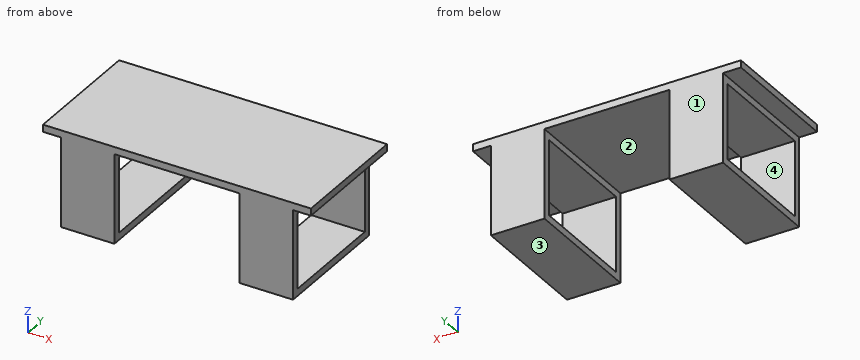
from build123d import *

# Parameters (mm, degrees)
F0_W     = 1500
F0_H     = 700
F1_DEPTH = 40
F2_W     = 300
F2_H     = 700
F3_DEPTH = 500
F4_W     = 620
F4_H     = 420
F5_DEPTH = 1328


with BuildPart() as f1:
    # F0 (on Top) → F1 (new body)
    with BuildSketch(Plane.XY):
        with Locations((750, -350)):
            Rectangle(F0_W, F0_H)
    extrude(amount=-F1_DEPTH)

    # F2 (on face) → F3 (join)
    with BuildSketch(Plane(origin=(0, 0, -40), x_dir=(1, 0, 0), z_dir=(0, 0, -1))):
        with Locations((250, 350)):
            Rectangle(F2_W, F2_H)
        with Locations((1250, 350)):
            Rectangle(F2_W, F2_H)
    extrude(amount=F3_DEPTH)

    # F4 (on face) → F5 (cut)
    with BuildSketch(Plane(origin=(100, 0, 0), x_dir=(0, -1, 0), z_dir=(-1, 0, 0))):
        with Locations((350, -290)):
            Rectangle(F4_W, F4_H)
    extrude(amount=-F5_DEPTH, mode=Mode.SUBTRACT)


solid = f1.part
Read the model definition and answer for the solid it produces. Units are mm, in the model's axes. Face numbers are marked on the shaded views. A direction names the side the tool comes from. Round coordinates to 2 decimals unless told otherwise and drop trailing zeros. Write each loop counter-clockwise with the first axis right and the second up, starting at its lowest first coordinate (ties: lowest second). Pieces come first, ordered by that corner, then holes. Notation, with made-up numbers: M 42,82.25 L 47,82.25 A25 ccw 47,95.25 Z; hole C -1,43.25 d1. An arc over 180 degrees is marked long. Use a Markdown table: item, result.
1) A flat-ended cylindrical pin translates along its axis: pin 1 (3 mm diameter, centred on x = 337, z = -308, fed in from +Y). Find the tip coordinate at first contact, or state that the pin passes through.
Answers follow:
| item | result |
|---|---|
| pin 1 | stops at y = 0 |
2) The part is cut by section C-C (y = -585). Write down the section's boundary in (x, z).
Answers follow:
| item | result |
|---|---|
| outline | M 0,-40 L 100,-40 L 100,-80 L 400,-80 L 400,-40 L 1100,-40 L 1100,-80 L 1400,-80 L 1400,-40 L 1500,-40 L 1500,0 L 0,0 Z; M 100,-540 L 400,-540 L 400,-500 L 100,-500 Z; M 1100,-540 L 1400,-540 L 1400,-500 L 1100,-500 Z |
3) The part is cut by section B-B (z = -245.5). Write down the section's boundary in (x, y), plus the area to 3 significant figures.
Answers follow:
| item | result |
|---|---|
| outline | M 100,-700 L 400,-700 L 400,-660 L 100,-660 Z; M 100,-40 L 400,-40 L 400,0 L 100,0 Z; M 1100,-700 L 1400,-700 L 1400,-660 L 1100,-660 Z; M 1100,-40 L 1400,-40 L 1400,0 L 1100,0 Z |
| area | 48,000 mm2 |
4) For a pull along X with two mould halves and no side action, classify the marked faces 1 and 2 as pulls with the +X half, pulls with the -X half, needs draft (parallel to the pull), parting line crosses it, or undercut.
Answers follow:
| item | result |
|---|---|
| face 1 | needs draft |
| face 2 | undercut |
5) Straight lines are drawn through the part: line 1 along Y through (x, z) = (133.5, -145.5); line 2 along Z through (x, y) = (1279.5, -317.5); line 3 along X through (y, z) = (-197.5, -57.5). For each, find the intervals that lie inside material, in ascending order. Write a range as [from, to].
Answers follow:
| item | result |
|---|---|
| line 1 | y = [-700, -660], [-40, 0] |
| line 2 | z = [-540, -500], [-80, 0] |
| line 3 | x = [100, 400], [1100, 1400] |
6) The part is cut by section A-A (x = 189.5). Write down the section's boundary in (y, z).
Answers follow:
| item | result |
|---|---|
| outline | M -700,-540 L 0,-540 L 0,0 L -700,0 Z; hole M -660,-500 L -40,-500 L -40,-80 L -660,-80 Z |
7) A tool of negligible diameter and unlimited length cuts with its end or side. For the marked faces 3 and 4, from which of +Z, -Z, +X, -X, +Y, -Y can it reach the whole face along a straight path? Write none if from no direction.
Answers follow:
| item | result |
|---|---|
| face 3 | -Z, +X, -X, +Y, -Y |
| face 4 | +X, -X |
8) The part is cut by section D-D (x = 552). Write down the section's boundary in (y, z), plus the area to 3 significant figures.
Answers follow:
| item | result |
|---|---|
| outline | M -700,-40 L 0,-40 L 0,0 L -700,0 Z |
| area | 28,000 mm2 |
